The model under review builds one solid part; all positions refer to its coordinate system, in mm. Coordinates: 2 decimals unless noted, no trailing zeros. Loops run counter-clockwise (first coordinate to the right, second up) from the corner with the lowest first, then second, coordinate; pieces in that order, holes last. Notation, with made-up numbers: M 36,65 L 55,65 A24 cw 55,99 Z; hole C -18.75,30 d5. An arc over 180 degrees is marked long. Use one line per item in the form item = value.
Autodesk Inventor part; units mm, degrees
ref_plane "YZ Plane" through (0, 0, 0) normal (1, 0, 0) x (0, 1, 0)
ref_plane "XZ Plane" through (0, 0, 0) normal (0, 1, 0) x (-1, 0, 0)
ref_plane "XY Plane" through (0, 0, 0) normal (0, 0, 1) x (1, 0, 0)
sketch "Sketch1" plane through (0, 0, 0) normal (0, 0, 1) x (1, 0, 0)
  line L0 (-11.8764, 47.9805) -> (133.1236, 47.9805)
  line L1 (133.1236, 47.9805) -> (135.6236, 50.4805)
  line L2 (135.6236, 50.4805) -> (135.6236, 55.4805)
  line L3 (135.6236, 55.4805) -> (133.1236, 57.9805)
  line L4 (133.1236, 57.9805) -> (75.6236, 57.9805)
  line L5 (-11.8764, 57.9805) -> (-14.3764, 55.4805)
  line L6 (-14.3764, 55.4805) -> (-14.3764, 50.4805)
  line L7 (-14.3764, 50.4805) -> (-11.8764, 47.9805)
  line L8 (75.6236, 57.9805) -> (75.6236, 67.9805)
  line L9 (75.6236, 67.9805) -> (65.6236, 77.9805)
  line L10 (65.6236, 77.9805) -> (55.6236, 77.9805)
  line L11 (55.6236, 77.9805) -> (45.6236, 67.9805)
  line L12 (45.6236, 67.9805) -> (45.6236, 57.9805)
  line L13 (45.6236, 57.9805) -> (-11.8764, 57.9805)
  circle A0 centre (-9.3764, 52.9805) radius 2
  circle A1 centre (130.6236, 52.9805) radius 2
  line L14 (200.7921, 30.8795) -> (340.7921, 30.8795) construction
  line L15 (245.7921, 30.8795) -> (245.7921, -89.1205) construction
  line L16 (198.2921, 35.8795) -> (343.2921, 35.8795)
  line L17 (240.7921, 5.8795) -> (240.7921, -91.6205)
  line L18 (250.7921, 5.8795) -> (250.7921, -91.6205)
  line L19 (248.2921, -94.1205) -> (243.2921, -94.1205)
  line L20 (195.7921, 33.3795) -> (195.7921, 28.3795)
  line L21 (345.7921, 33.3795) -> (345.7921, 28.3795)
  line L22 (240.7921, -91.6205) -> (243.2921, -94.1205)
  line L23 (250.7921, -91.6205) -> (248.2921, -94.1205)
  line L24 (343.2921, 25.8795) -> (345.7921, 28.3795)
  line L25 (345.7921, 33.3795) -> (343.2921, 35.8795)
  line L26 (198.2921, 35.8795) -> (195.7921, 33.3795)
  line L27 (195.7921, 28.3795) -> (198.2921, 25.8795)
  line L28 (198.2921, 25.8795) -> (230.7921, 25.8795)
  line L29 (260.7921, 25.8795) -> (343.2921, 25.8795)
  line L30 (260.7921, 25.8795) -> (260.7921, 15.8795)
  line L31 (230.7921, 15.8795) -> (230.7921, 25.8795)
  line L32 (250.7921, 5.8795) -> (260.7921, 15.8795)
  line L33 (240.7921, 5.8795) -> (230.7921, 15.8795)
  point P0 (195.7921, 35.8795)
  point P1 (345.7921, 35.8795)
  point P2 (195.7921, 25.8795)
  point P3 (345.7921, 25.8795)
  point P4 (240.7921, -94.1205)
  point P5 (250.7921, -94.1205)
  point P6 (260.7921, 5.8795)
  point P7 (230.7921, 5.8795)
  dimension "d54" = 140
  dimension "d55" = 120
  dimension "d56" = 45
  dimension "d57" = 5
  dimension "d59" = 5
  dimension "d60" = 5
  dimension "d61" = 5
  dimension "d62" = 5
  dimension "d63" = 5
  dimension "d64" = 2.5
  dimension "d65" = 2.5
  dimension "d66" = 2.5
  dimension "d67" = 2.5
  dimension "d68" = 2.5
  dimension "d69" = 2.5
  dimension "d70" = 2.5
  dimension "d71" = 2.5
  dimension "d72" = 2.5
  dimension "d73" = 2.5
  dimension "d74" = 2.5
  dimension "d75" = 2.5
  dimension "d76" = 30
  dimension "d77" = 20
  dimension "d78" = 15
  dimension "d79" = 10
  dimension "d80" = 10
  dimension "d81" = 10
  dimension "d82" = 10
extrude "Extrusion1" add sketch "Sketch1" along normal blind 7 contours L16 L25 L21 L24 L29 L30 L32 L18 L23 L19 L22 L17 L33 L31 L28 L27 L20 L26
sketch "Sketch2" plane through (0, 0, 7) normal (0, 0, 1) x (1, 0, 0)
  line L0 (195.7921, 33.3795) -> (195.7921, 28.3795)
  line L1 (345.7921, 28.3795) -> (345.7921, 33.3795)
  point P0 (200.7921, 30.8795)
  point P1 (340.7921, 30.8795)
  dimension "d83" = 5
  dimension "d84" = 5
hole "Hole1" at (200.7921, 30.8795, 7) at (340.7921, 30.8795, 7) direction (0, 0, -1) diameter 4 end through all
sketch "Sketch4" plane through (0, 0, 7) normal (0, 0, 1) x (1, 0, 0)
  circle A0 centre (200.7921, 30.8795) radius 2 construction
  circle A1 centre (340.7921, 30.8795) radius 2 construction
  line L0 (200.7921, 30.8795) -> (340.7921, 30.8795) construction
  line L1 (245.7921, -89.1205) -> (245.7921, 30.8795) construction
  line L2 (243.2921, -94.1205) -> (248.2921, -94.1205) construction
  line L3 (243.7921, -89.1205) -> (243.7921, 0.8795)
  line L4 (247.7921, 0.8795) -> (247.7921, -89.1205)
  arc A2 (247.7921, 0.8795) -> (243.7921, 0.8795) centre (245.7921, 0.8795) ccw
  arc A3 (243.7921, -89.1205) -> (247.7921, -89.1205) centre (245.7921, -89.1205) ccw
  point P0 (0, 0)
  point P1 (245.7921, -94.1205)
  dimension "d89" = 2
  dimension "d90" = 45
  dimension "d92" = 5
  dimension "d93" = 2
extrude "Extrusion3" cut sketch "Sketch4" against normal blind 7
properties part number "tLever" material "MDF Medium Density Fiberboard"
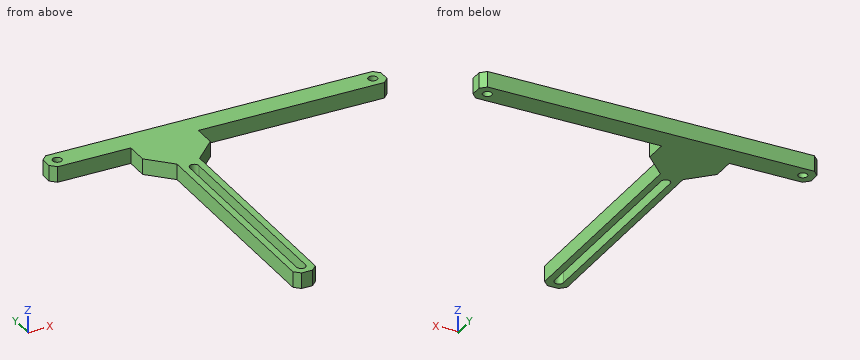
1. Add section C-C (y = 20). State the section outline as (x, z) points.
Response values:
outline = M 230.79,0 L 260.79,0 L 260.79,7 L 230.79,7 Z
2. Add section A-A (y = -62). State the section outline as (x, z) points.
Response values:
outline = M 240.79,0 L 243.79,0 L 243.79,7 L 240.79,7 Z; M 247.79,0 L 250.79,0 L 250.79,7 L 247.79,7 Z
3. Wall thickness on line 1 along X through (y, z) = (-70.5, 1); line 2 along Y through (x, z) = (290, 5.5); line 3 along X through (y, z) = (1.5, 4.5): over which ranges is each line inside the solid? List them lowest first. Write a range as from..to.
Response values:
line_1 = 240.79..243.79, 247.79..250.79
line_2 = 25.88..35.88
line_3 = 240.79..243.89, 247.69..250.79
4. Add section D-D (x = 271). State the section outline as (y, z) points, then the cut area to 3 significant figures.
Response values:
outline = M 25.88,0 L 35.88,0 L 35.88,7 L 25.88,7 Z
area = 70.0 mm^2
5. Add section B-B (z = 3). State the section outline as (x, y) points, then the cut area to 3 significant figures.
Response values:
outline = M 195.79,28.38 L 198.29,25.88 L 230.79,25.88 L 230.79,15.88 L 240.79,5.88 L 240.79,-91.62 L 243.29,-94.12 L 248.29,-94.12 L 250.79,-91.62 L 250.79,5.88 L 260.79,15.88 L 260.79,25.88 L 343.29,25.88 L 345.79,28.38 L 345.79,33.38 L 343.29,35.88 L 198.29,35.88 L 195.79,33.38 Z; hole C 200.79,30.88 d4; hole M 243.79,-89.12 A2 ccw 247.79,-89.12 L 247.79,0.88 A2 ccw 243.79,0.88 Z; hole C 340.79,30.88 d4
area = 2,580 mm^2
6. Insertion check: P1, Ø3.5, axis at y = -38, z = 2, coming from the +X side; P2, Ø2, axis at y = -25, z = 2, coming from the -X side; P3, Ø3.5, axis at x = 211.5, z = 5, coming from the -Y side. Each pin has a flat end and moves straight along its axis. Give the tip position at first contact, or say it passes through.
Response values:
P1 = 250.79
P2 = 240.79
P3 = 25.88
